from build123d import *
from build123d import SkipClean  # not in build123d's __all__

# Parameters (mm, degrees)
F1_DEPTH      = 5
F2_R          = 2.5
F3_DEPTH      = 1
F4_SIZE       = 0.99999
F5_R          = 2.5
F6_DEPTH      = 1
F7_SIZE       = 0.99999
F8_R          = 2.4999
F9_R          = 4.5
F10_DEPTH     = 10
F11_T1_DEPTH  = 5.5001
F11_T3_DEPTH  = 0.0002
F11_T6_ANGLE  = 90
F11_T8_ANGLE  = 90
F11_T10_ANGLE = 90
F11_T12_ANGLE = 90


# Not quite as in the source:
# - a fillet or chamfer that OpenCascade refuses, or shapes differently, is made with other operations: its cross-section is extruded or revolved along the edge and cut away or added
# - a fillet or chamfer is up to 0.001 mm smaller than in the source, because OpenCascade refuses the exact size


with BuildPart() as f1:
    # F0 (on Top) → F1 (new body)
    with BuildSketch(Plane.XY):
        Polygon((15.446737438, 4.2690986316), (10.446737438, 4.2690986316), (10.446737438, 10.2690986316), (8.446737438, 10.2690986316), (8.446737438, 2.2690986316), (17.446737438, 2.2690986316), (17.446737438, 10.2690986316), (15.446737438, 10.2690986316), align=None)
    extrude(amount=F1_DEPTH)

    # F2 (on face) → F3 (join)
    with BuildSketch(Plane.YZ.offset(10.446737438)):
        with Locations((7.7690986316, 2.5)):
            Circle(F2_R)
    extrude(amount=F3_DEPTH)

    # F4 (size 1 in the source; OpenCascade refuses exactly that, so slightly less here)
    f4_edges = [f1.edges().sort_by_distance(p)[0] for p in [
        (11.446737, 5.269099, 2.5),
    ]]
    chamfer(f4_edges, length=F4_SIZE)

    # F5 (on face) → F6 (join)
    with BuildSketch(Plane(origin=(15.446737438, 0, 0), x_dir=(0, -1, 0), z_dir=(-1, 0, 0))):
        with Locations((-7.7690986316, 2.5)):
            Circle(F5_R)
    extrude(amount=F6_DEPTH)

    # F7 (size 1 in the source; OpenCascade refuses exactly that, so slightly less here)
    f7_edges = [f1.edges().sort_by_distance(p)[0] for p in [
        (14.446737, 10.269099, 2.5),
    ]]
    chamfer(f7_edges, length=F7_SIZE)

    # F8 (radius 2.5 in the source; OpenCascade refuses exactly that, so slightly less here)
    f8_edges = [f1.edges().sort_by_distance(p)[0] for p in [
        (16.446737, 10.269099, 5),
        (16.446737, 10.269099, 0),
        (9.446737, 10.269099, 5),
        (9.446737, 10.269099, 0),
    ]]
    fillet(f8_edges, radius=F8_R)

    # F9 (on face) → F10 (join)
    with BuildSketch(Plane.XZ.offset(-2.2690986316)):
        with Locations((12.946737438, 2.5)):
            Circle(F9_R)
    extrude(amount=F10_DEPTH)

    # F11: fillet of radius 2 on 4 edges, made by hand

    # F11_s2 → F11_t1 (cut)
    with BuildSketch(Plane.XZ.offset(-7.7691986316)):
        with BuildLine():
            ThreePointArc((8.446737438, 3), (9.0325238756, 4.4142135624), (10.446737438, 5))
            Line((10.446737438, 5), (8.446737438, 5))
            Line((8.446737438, 5), (8.446737438, 3))
        make_face()
        with BuildLine():
            ThreePointArc((10.446737438, 0), (9.0325238756, 0.5857864376), (8.446737438, 2))
            Line((8.446737438, 2), (8.446737438, 0))
            Line((8.446737438, 0), (10.446737438, 0))
        make_face()
        with BuildLine():
            ThreePointArc((15.446737438, 0), (16.8609510003, 0.5857864376), (17.446737438, 2))
            Line((17.446737438, 2), (17.446737438, 0))
            Line((17.446737438, 0), (15.446737438, 0))
        make_face()
        with BuildLine():
            ThreePointArc((17.446737438, 3), (16.8609510003, 4.4142135624), (15.446737438, 5))
            Line((15.446737438, 5), (17.446737438, 5))
            Line((17.446737438, 5), (17.446737438, 3))
        make_face()
    extrude(amount=F11_T1_DEPTH, mode=Mode.SUBTRACT)

    # F11_s4 → F11_t3 (cut)
    with BuildSketch(Plane.XY.offset(2.4999)):
        with BuildLine():
            ThreePointArc((15.446737438, 10.2690986316), (16.8609510003, 9.6833121939), (17.446737438, 8.2690986316))
            Line((17.446737438, 8.2690986316), (17.446737438, 10.2690986316))
            Line((17.446737438, 10.2690986316), (15.446737438, 10.2690986316))
        make_face()
        with BuildLine():
            ThreePointArc((8.446737438, 8.2690986316), (9.0325238756, 9.6833121939), (10.446737438, 10.2690986316))
            Line((10.446737438, 10.2690986316), (8.446737438, 10.2690986316))
            Line((8.446737438, 10.2690986316), (8.446737438, 8.2690986316))
        make_face()
    with SkipClean():  # cleaning this boolean's faces spoils the solid; the shape is the same uncleaned
        extrude(amount=F11_T3_DEPTH, mode=Mode.SUBTRACT)

    # F11_s5 → F11_t6 (revolve, cut)
    with BuildSketch(Plane.XZ.offset(-7.7691986316)):
        with BuildLine():
            ThreePointArc((17.446737438, 3), (16.8609510003, 4.4142135624), (15.446737438, 5))
            Line((15.446737438, 5), (17.446737438, 5))
            Line((17.446737438, 5), (17.446737438, 3))
        make_face()
    with SkipClean():  # cleaning this boolean's faces spoils the solid; the shape is the same uncleaned
        revolve(axis=Axis((17.446737438, 7.7691986316, 2.5001), (-1, 0, 0)), revolution_arc=F11_T6_ANGLE, mode=Mode.SUBTRACT)

    # F11_s7 → F11_t8 (revolve, cut)
    with BuildSketch(Plane.XZ.offset(-7.7691986316)):
        with BuildLine():
            ThreePointArc((15.446737438, 0), (16.8609510003, 0.5857864376), (17.446737438, 2))
            Line((17.446737438, 2), (17.446737438, 0))
            Line((17.446737438, 0), (15.446737438, 0))
        make_face()
    with SkipClean():  # cleaning this boolean's faces spoils the solid; the shape is the same uncleaned
        revolve(axis=Axis((17.446737438, 7.7691986316, 2.4999), (1, 0, 0)), revolution_arc=F11_T8_ANGLE, mode=Mode.SUBTRACT)

    # F11_s9 → F11_t10 (revolve, cut)
    with BuildSketch(Plane.XZ.offset(-7.7691986316)):
        with BuildLine():
            ThreePointArc((10.446737438, 0), (9.0325238756, 0.5857864376), (8.446737438, 2))
            Line((8.446737438, 2), (8.446737438, 0))
            Line((8.446737438, 0), (10.446737438, 0))
        make_face()
    revolve(axis=Axis((8.446737438, 7.7691986316, 2.4999), (1, 0, 0)), revolution_arc=F11_T10_ANGLE, mode=Mode.SUBTRACT)

    # F11_s11 → F11_t12 (revolve, cut)
    with BuildSketch(Plane.XZ.offset(-7.7691986316)):
        with BuildLine():
            ThreePointArc((8.446737438, 3), (9.0325238756, 4.4142135624), (10.446737438, 5))
            Line((10.446737438, 5), (8.446737438, 5))
            Line((8.446737438, 5), (8.446737438, 3))
        make_face()
    revolve(axis=Axis((8.446737438, 7.7691986316, 2.5001), (-1, 0, 0)), revolution_arc=F11_T12_ANGLE, mode=Mode.SUBTRACT)


solid = f1.part
Design review of the part built by this model. Coordinates are the model's own, in mm. A direction names the side the tool comes from. Give positions to 0.01 mm unless a question says otherwise; leave off trailing zeros. Order: outer loops, then holes, each group sorted by start corner. A loop starts at its lowest first (then second) coordinate and runs counter-clockwise, first axis right, second up.
1. Add section A-A, the plane y = 4.75. State the section outline as (x, z) points.
Solution:
outline: (8.45, 2) arc R2 ccw to (10.45, 0) - (10.45, 5) arc R2 ccw to (8.45, 3) - close; (15.45, 0) arc R2 ccw to (17.45, 2) - (17.45, 3) arc R2 ccw to (15.45, 5) - close
2. For pin 1 Ø2 at (y, z) = (9, 3.5) entering from +X; pin 2 Ø2 at (y, z) = (7.5, 4.5) entering from -X; pin 3 Ø3.5 at (x, z) = (12.5, -1) entering from +Y, all flat-tipped, find the tip position at first contact; note any pin that passes through.
Solution:
pin 1: stops at x = 17.44
pin 2: stops at x = 8.51
pin 3: stops at y = 4.27
3. Mouldability with a two-part tool opening along Y and no side actions: class faces 1 (the flat face through (14.447, 8, 3)), 2 (the flat face through (15.447, 5, 2)), 3 (the flat face through (13, 2.269, 6)) as +Y half, -Y half, draft (parallel to the pull), parting line (faces both ways), or undercut.
Solution:
face 1: draft
face 2: undercut
face 3: +Y half
4. Add section C-C, the plane z = 5.5. State the section outline as (x, y) points, then the cut area to 3 significant figures.
Solution:
outline: (9.59, -7.73) - (16.3, -7.73) - (16.3, 2.27) - (9.59, 2.27) - close
area: 67.1 mm2
5. To check wall thickness, follow L1, parallel to Y at x = 12.5, z = 6; L2, parallel to Y at x = 11.5, z = 1.25; L3, parallel to X at y = 5.5, z = 0.25. State the ranges of each line that lie inside material, in increasing order.
Solution:
L1: y = -7.73 to 2.27
L2: y = -7.73 to 4.27
L3: x = 9.48 to 10.45, 15.45 to 16.41
6. Tool access review of faces 4 (the flat face through (13, 4.269, 2)), 5 (the cylindrical face through (8.45, -2.66, 2.7)), 6 (the flat face through (13, 3, 0)), 7 (the flat face through (11.447, 8, 3)): name each direction out of +Z, -Z, +X, -X, +Y, -Y from which nothing blocks a thin tool from reaching the whole face with its end or side.
Solution:
face 4: +Z, -Z
face 5: -Y
face 6: -Z, +X, -X, +Y
face 7: +Z, -Z, +Y
7. Add section B-B, the plane x = 13.25. State the section outline as (y, z) points, then the cut area to 3 significant figures.
Solution:
outline: (-7.73, -1.99) - (2.27, -1.99) - (2.27, 0) - (4.27, 0) - (4.27, 5) - (2.27, 5) - (2.27, 6.99) - (-7.73, 6.99) - close
area: 99.8 mm2
8. Add section D-D, the plane y = -3. State the section outline as (x, z) points, then the cut area to 3 significant figures.
Solution:
outline: circle Ø9 at (12.95, 2.5)
area: 63.6 mm2
